Verification items for this drawing (mm, ordinates from the low corner). A direction names the side the tool comes from. Coordinates: 2 decimals unless noted, no trailing zeros. Order: outer loops, then holes, each group sorted by start corner. A loop starts at its lowest first (then second) coordinate and runs counter-clockwise, first axis right, second up. Notation, with made-up numbers: (8, 9) -> (12, 9) arc R28 cw to (12, 47) -> close; hole circle Ø6 at (-39, -32.75). An arc over 180 degrees is marked (long way). Write each question's results on one line, items separated by ' | '. Start each with the question number.
(1) Thickness scan on probe 1 along Y at (x, z) = (14.5, 7.75); probe 2 along Y at (x, z) = (22.75, 24); probe 3 along Y at (x, z) = (22, 14.25). Record the ranges inside material, lowest first. Write a range as [from, to].
(2) Set-up check for the marked faces 1, 2 and 3: record each of +Z, -Z, +X, -X, +Y, -Y from which the full face is reachable in a straight line by a thin tool's end or side.
(3) Cross-section at D-D on z = 3.5. Enter the section's corners in (x, y).
(4) Cross-section at C-C on y = 4. Enter the section's corners in (x, z), and give its area (3 significant figures).
(5) Cross-section at B-B on x = 8.5. Enter the section's corners in (y, z), and give its area (3 significant figures).
(6) Go/stop test with flat-tipped pins: pin 1 (7.5 mm diameter, centred on x = 9.5, y = 3, fed in from +Z); pin 2 (1.5 mm diameter, centred on x = 3.5, y = 10, fed in from +Z); pin 3 (0.6 mm diameter, centred on x = 18.5, y = 15, fed in from +Z); pin 4 (5 mm diameter, centred on x = 17.5, z = 11, fed in from +Y). Record where each tip stops, or that it passes through.
(7) Cross-section at A-A on z = 22.75. Enter the section's corners in (x, y), and give its area (3 significant figures).
(8) Draft check along Y on the marked faces 4, 5 and 6. Enter one of: +Y half, -Y half, draft (parallel to the pull), parting line (faces both ways), or undercut.
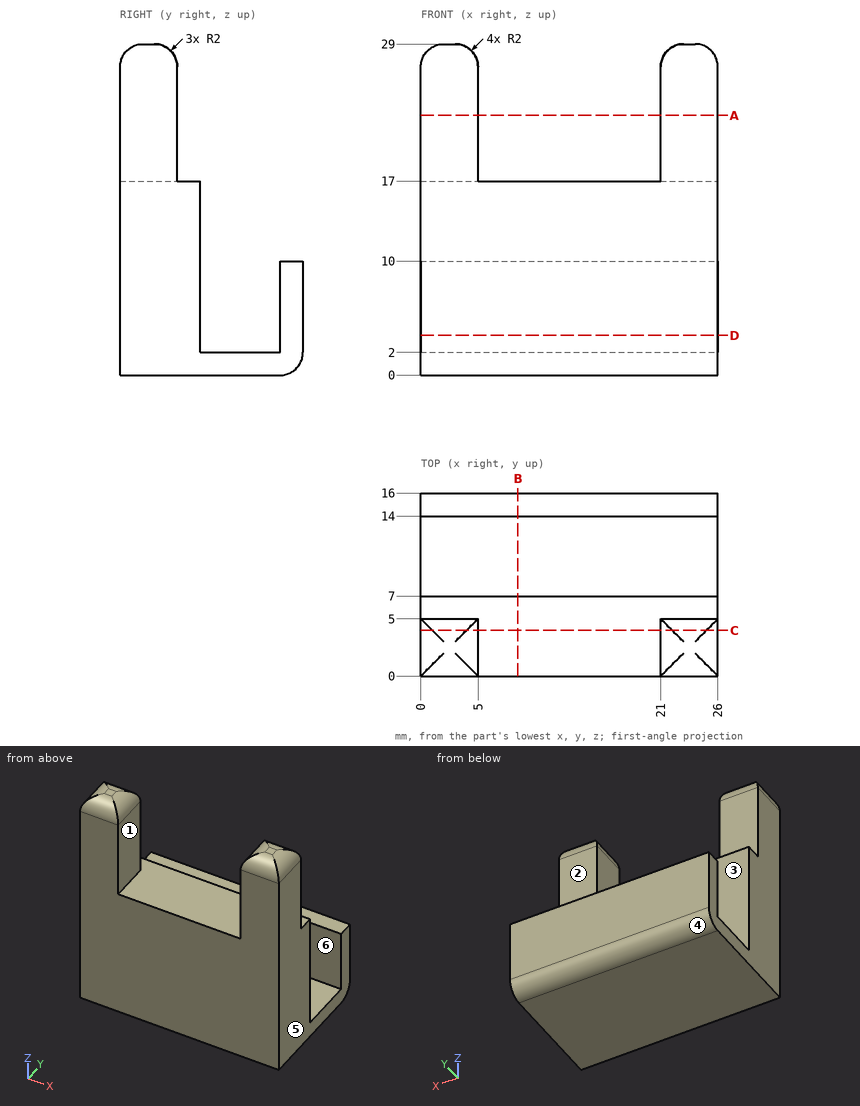
Results are:
1) probe 1: y = [0, 7], [14, 16] | probe 2: y = [0, 5] | probe 3: y = [0, 7]
2) face 1: +Z, +Y, -Y | face 2: +Z, +X, -X, +Y | face 3: +Z, +X, -X
3) outline: (0, 0) -> (26, 0) -> (26, 7) -> (0, 7) -> close; (0, 14) -> (26, 14) -> (26, 16) -> (0, 16) -> close
4) outline: (0, 0) -> (26, 0) -> (26, 27) arc R2 ccw to (25, 28.73) -> (22, 28.73) arc R2 ccw to (21, 27) -> (21, 17) -> (5, 17) -> (5, 27) arc R2 ccw to (4, 28.73) -> (1, 28.73) arc R2 ccw to (0, 27) -> close | area: 557 mm2
5) outline: (0, 0) -> (14, 0) arc R2 ccw to (16, 2) -> (16, 10) -> (14, 10) -> (14, 2) -> (7, 2) -> (7, 17) -> (0, 17) -> close | area: 152 mm2
6) pin 1: stops at z = 17 | pin 2: stops at z = 2 | pin 3: stops at z = 10 | pin 4: stops at y = 16
7) outline: (0, 0) -> (5, 0) -> (5, 5) -> (0, 5) -> close; (21, 0) -> (26, 0) -> (26, 5) -> (21, 5) -> close | area: 50.0 mm2
8) face 4: +Y half | face 5: draft | face 6: undercut
